```python
from build123d import *

# Parameters (mm, degrees)
F1_DEPTH = 25.4
F2_R     = 7.488369
F3_DEPTH = 12.7


with BuildPart() as f1:
    # F0 (on Right) → F1 (new body)
    with BuildSketch(Plane.YZ):
        Polygon((19.569545, -43.848365), (47.749595, 5.061853), (9.941328, 46.976762), (-41.605517, 23.971383), (-35.654951, -32.161633), align=None)
    extrude(amount=F1_DEPTH)

    # F2 (on face) → F3 (join)
    with BuildSketch(Plane(origin=(0, 0, 0), x_dir=(0, -1, 0), z_dir=(-1, 0, 0))):
        Circle(F2_R)
    extrude(amount=F3_DEPTH)


solid = f1.part
```
Input: part model. Units: mm. Frame: model coordinates. A direction names the side the tool comes from. Coordinates: 2 decimals unless noted, no trailing zeros. Loops run counter-clockwise (first coordinate to the right, second up) from the corner with the lowest first, then second, coordinate; pieces in that order, holes last. Notation, with made-up numbers: (56.25, 84) -> (113.25, 84) arc R10 ccw to (113.25, 101) -> close; hole circle Ø9 at (-0.75, 0). An arc over 180 degrees is marked (long way). Use a Markdown table: item, result.
1) Cut plane C-C (x = -10). Return the cut outline in (y, z).
Results found:
| item | result |
|---|---|
| outline | circle Ø14.98 at (0, 0) |
2) Material intervals for line 1 along X through (y, z) = (15, -10.5); line 2 along Y through (x, z) = (2, 22); line 3 along Z through (x, y) = (-5, -6.5), sorted ascending. Write a range as from..to.
Results found:
| item | result |
|---|---|
| line 1 | x = 0..25.4 |
| line 2 | y = -41.4..32.47 |
| line 3 | z = -3.72..3.72 |
3) Cut plane D-D (z = -15). Return the cut outline in (x, y).
Results found:
| item | result |
|---|---|
| outline | (0, -37.47) -> (25.4, -37.47) -> (25.4, 36.19) -> (0, 36.19) -> close |
4) Contact query for flat-ended pins moving along their axis: pin 1 (12 mm diameter, centred on x = 2, y = 29.5, fed in from +Z); pin 2 (5 mm diameter, centred on x = 12, y = 8.5, fed in from -Z); pin 3 (6 mm diameter, centred on x = 0, y = -23, fed in from +Z). Output: stop coordinate, or through.
Results found:
| item | result |
|---|---|
| pin 1 | stops at z = 31.95 |
| pin 2 | stops at z = -42.03 |
| pin 3 | stops at z = 33.61 |
5) Cut plane A-A (z = 0). Return the cut outline in (x, y).
Results found:
| item | result |
|---|---|
| outline | (-12.7, -7.49) -> (0, -7.49) -> (0, -39.06) -> (25.4, -39.06) -> (25.4, 44.83) -> (0, 44.83) -> (0, 7.49) -> (-12.7, 7.49) -> close |
6) Cut plane B-B (y = 0). Return the cut outline in (x, z).
Results found:
| item | result |
|---|---|
| outline | (-12.7, -7.49) -> (0, -7.49) -> (0, -39.71) -> (25.4, -39.71) -> (25.4, 42.54) -> (0, 42.54) -> (0, 7.49) -> (-12.7, 7.49) -> close |
7) Access query for faces 1 (the flat face through (12.52, 33.46, -19.74)), 2 (the cylindrical face through (-6.261, 0.975, 7.425)). Directions: +Z, -Z, +X, -X, +Y, -Y. A direction counts if a zero-diameter tool reaches every point of the face in a straight line with its end or side. Return the directions, or none.
Results found:
| item | result |
|---|---|
| face 1 | -Z, +X, -X, +Y |
| face 2 | -X |
